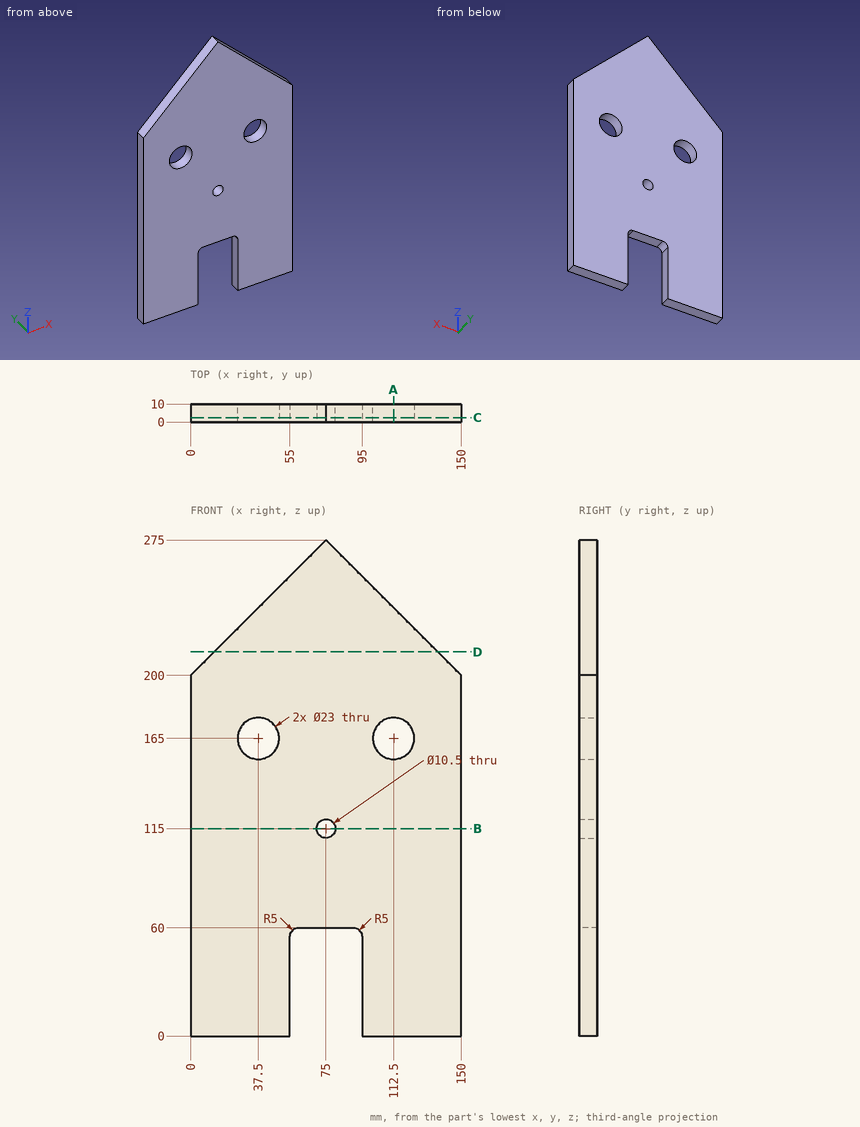
Drawing for the job (mm, zero at the part's lowest x, y, z). Round coordinates to 2 decimals unless told otherwise and drop trailing zeros. Loops run counter-clockwise (first coordinate to the right, second up) from the corner with the lowest first, then second, coordinate; pieces in that order, holes last. Notation, with made-up numbers: M -4.75,69.25 L 28.25,69.25 A26 ccw 28.25,86.25 Z; hole C -23,75.5 d4. An arc over 180 degrees is marked long. Use a Markdown table: item, result. Add a question column.
(1) Cut at D-D (z = 213). Give the cut face in (x, y), and give its area (3 significant figures).
(2) Flat gauge pins, fed straight in: pin 1 (13.5 mm diameter, centred on x = 75, z = 115, fed in from +Y); pin 2 (5 mm diameter, centred on x = 68.5, y = 4, fed in from -Z); pin 3 (4 mm diameter, centred on y = 1.5, z = 202.5, fed in from +X). Where does each tip first touch, or does it go through?
(3) Drill centre lines: line 1 (X direction, y = 9, z = 45); line 2 (X direction, y = 2.5, z = 157.5); line 3 (X direction, y = 5.5, z = 156.5). Where is each one in solid material? Low to high.
(4) Cut at A-A (x = 112.5). Give the cut face in (y, z).
(5) Cut at B-B (z = 115). Give the cut face in (x, y).
(6) Cut at C-C (y = 2.5). Give the cut face in (x, z), and give its area (3 significant figures).
Geometry says:
| question | item | result |
|---|---|---|
| 1 | outline | M 13,0 L 137,0 L 137,10 L 13,10 Z |
| 1 | area | 1,240 mm² |
| 2 | pin 1 | stops at y = 10 |
| 2 | pin 2 | stops at z = 60 |
| 2 | pin 3 | stops at x = 149.5 |
| 3 | line 1 | x = 0 to 55, 95 to 150 |
| 3 | line 2 | x = 0 to 28.78, 46.22 to 103.78, 121.22 to 150 |
| 3 | line 3 | x = 0 to 29.75, 45.25 to 104.75, 120.25 to 150 |
| 4 | outline | M 0,0 L 10,0 L 10,153.5 L 0,153.5 Z; M 0,176.5 L 10,176.5 L 10,237.5 L 0,237.5 Z |
| 5 | outline | M 0,0 L 69.75,0 L 69.75,10 L 0,10 Z; M 80.25,0 L 150,0 L 150,10 L 80.25,10 Z |
| 6 | outline | M 0,0 L 55,0 L 55,55 A5 cw 60,60 L 90,60 A5 cw 95,55 L 95,0 L 150,0 L 150,200 L 75,275 L 0,200 Z; hole C 37.5,165 d23; hole C 75,115 d10.5; hole C 112.5,165 d23 |
| 6 | area | 32,300 mm² |
